The figure shows three views and two pictorial views of one solid part (mm, origin at its lowest corner). Answer the questions. A direction names the side the tool comes from. Round coordinates to 2 decimals unless told otherwise and drop trailing zeros. Loops run counter-clockwise (first coordinate to the right, second up) from the corner with the lowest first, then second, coordinate; pieces in that order, holes last. Notation, with made-up numbers: (-21, -28.5) -> (8, -28.5) arc R27 ccw to (8, -5.5) -> close; hole circle Ø8 at (-25, 5). An arc over 180 degrees is marked (long way). Write item = value, one per line. Start each with the question number.
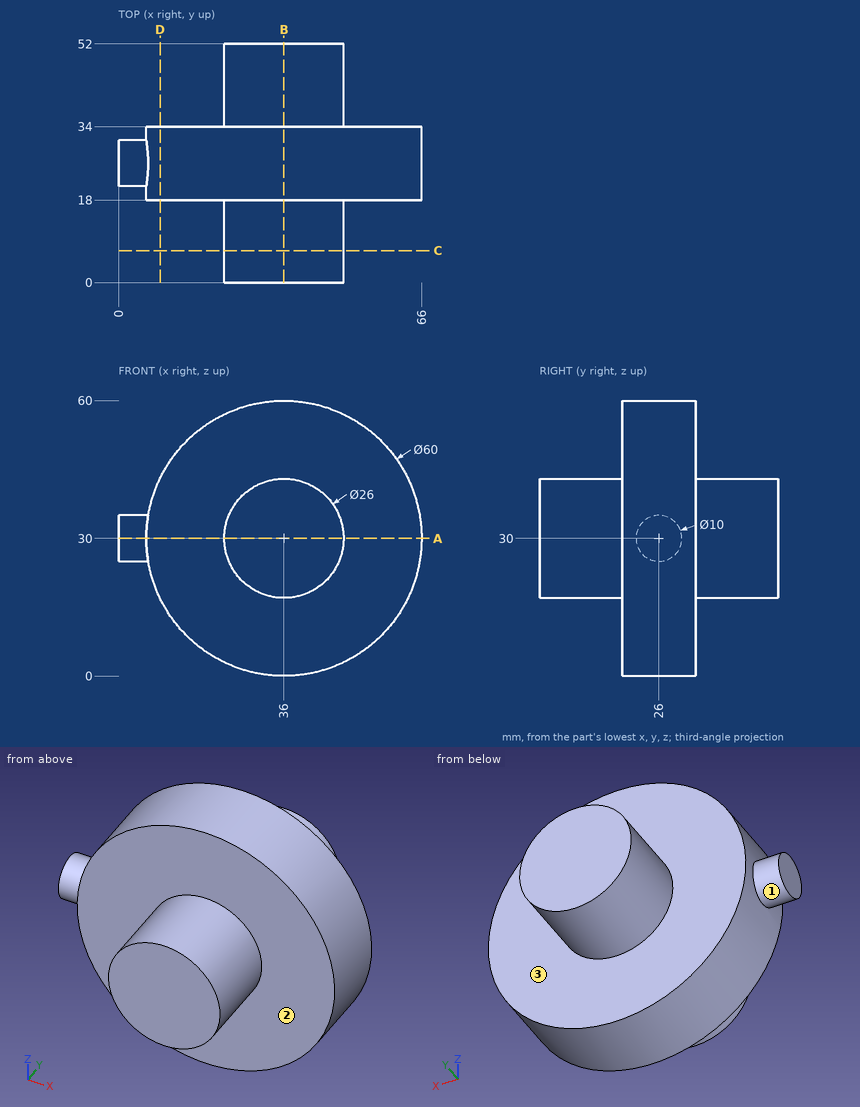
Item 1: Section C-C (y = 7) is taken. Determine the outline of the cut face in (x, z), then the cut area to 3 significant figures.
Item 2: Section B-B (x = 36) is taken. Determine the outline of the cut face in (y, z), then the cut area to 3 significant figures.
Item 3: Find the intervals of material crossed by line 1 along Y through (x, z) = (42, 15); line 2 along Z through (x, y) = (28.5, 22); line 3 along Z through (x, y) = (23, 33.5), in increasing order. Write a range as [from, to].
Item 4: Section D-D (x = 9) is taken. Determine the outline of the cut face in (y, z).
Item 5: Flat-ended cylindrical pins translate along their axes: pin 1 (5 mm diameter, centred on y = 44.5, z = 31, fed in from -X); pin 2 (6 mm diameter, centred on x = 32.5, z = 47, fed in from -Y); pin 3 (5 mm diameter, centred on y = 17.5, z = 50.5, fed in from -X). Find the tip coordinate at first contact, or state that the pin passes through.
Item 6: A tool of negligible diameter and unlimited length cuts with its end or side. For the marked faces 1, 2 and 3, from which of +Z, -Z, +X, -X, +Y, -Y can it reach the whole face along a straight path? Write none if from no direction.
Item 7: Section A-A (z = 30) is taken. Determine the outline of the cut face in (x, y).
Worked answers:
q1.outline = circle Ø26 at (36, 30)
q1.area = 531 mm2
q2.outline = (0, 17) -> (18, 17) -> (18, 0) -> (34, 0) -> (34, 17) -> (52, 17) -> (52, 43) -> (34, 43) -> (34, 60) -> (18, 60) -> (18, 43) -> (0, 43) -> close
q2.area = 1,900 mm2
q3.line_1 = [18, 34]
q3.line_2 = [0.95, 59.05]
q3.line_3 = [2.96, 57.04]
q4.outline = (18, 16.92) -> (34, 16.92) -> (34, 43.08) -> (18, 43.08) -> close
q5.pin_1 = 23
q5.pin_2 = 18
q5.pin_3 = 12.04
q6.face_1 = -X
q6.face_2 = -Y
q6.face_3 = +Y
q7.outline = (0, 21) -> (6, 21) -> (6, 18) -> (23, 18) -> (23, 0) -> (49, 0) -> (49, 18) -> (66, 18) -> (66, 34) -> (49, 34) -> (49, 52) -> (23, 52) -> (23, 34) -> (6, 34) -> (6, 31) -> (0, 31) -> close
